The listing builds one solid part. Answer for the finished solid, in the listing's coordinates (mm). A direction names the side the tool comes from. Give positions to 0.01 mm unless a question says otherwise; leave off trailing zeros. Order: outer loops, then holes, each group sorted by start corner. A loop starts at its lowest first (then second) coordinate and runs counter-clockwise, first axis right, second up. Notation, with made-up numbers: (-32, -37.75) - (5, -37.75) arc R23 cw to (5, -18.75) - close; hole circle Ø11 at (45.25, -35.5). An arc over 180 degrees is marked (long way). Answer as a JSON object with one key per item and string values. Group by question number.
Q1. The mould has two halves that part along X. Classify faces 5 (the face through (-10.084, 0.105, 17.68)), 6 (the face through (0.094, -0.424, 11.241)), 7 (the face through (0.588, 9.755, 18.163)): released by +X, released by -X, zero draft, split by the parting line, or undercut.
Q2. A cutting plane is placed at D-D, the plane x = 3.5. Give the vertices of the cut face in (y, z), and give its area (3 significant figures).
Q3. For faces 1 (the face through (12.34, 0.1, 48.11)), 2 (the face through (-8.5, 0, 5)), 3 (the face through (-0.531, 17.36, 20.162)), 4 (the face through (8.5, 0, 5)), determine the directions among +Z, -Z, +X, -X, +Y, -Y from which every point of the face is accessible in a straight line to the end or side of a thin tool.
Q4. A cutting plane is placed at C-C, the plane z = 22.5. Give the vertices of the cut face in (x, y).
Q5. A cutting plane is placed at A-A, the plane z = 33. Give the vertices of the cut face in (x, y).
Q6. Given pin 1 (7 mm diameter, centred on y = 2.5, z = 7, fed in from -X); pin 2 (8.5 mm diameter, centred on x = -4.5, z = 33.5, fed in from +Y); pin 3 (1 mm diameter, centred on x = -6.5, y = 17, fed in from -Z); pin 4 (10 mm diameter, centred on y = -3, z = 4, fed in from +X), each flat-ended and moving along its own axis, determine where each tip first touches the part or whether it passes through.
Q7. Consider line 1 (Y direction, x = 0, z = 3); line 2 (X direction, y = -4, z = 39); line 3 (X direction, y = 25, z = 38). Determine where each line is inside the solid, lowest interval first.
from build123d import *

# Parameters (mm, degrees)
ESQUISSE1_W                    = 17
ESQUISSE1_H                    = 15
BOSS_EXTRU_1_DEPTH             = 20
TROUS_DE_CENTRAGE_5_0MM1_D     = 5
TROUS_DE_CENTRAGE_5_0MM1_DEPTH = 10
TROUS_DE_CENTRAGE_5_0MM1_TIP   = 1.5021515475689007
BOSS_EXTRU_2_DEPTH             = 20
BOSS_EXTRU_3_START             = 15
BOSS_EXTRU_3_DEPTH             = 15
CONG_1_R                       = 19.999999999999996
CONG_2_R                       = 1


with BuildPart() as part:
    # Esquisse1 → Boss.-Extru.1 (new body)
    with BuildSketch(Plane.XY):
        Rectangle(ESQUISSE1_W, ESQUISSE1_H)
    extrude(amount=BOSS_EXTRU_1_DEPTH)

    # Trous de centrage Ø5.0mm1
    with Locations(Plane(origin=(0, 0, 0), x_dir=(-1, 0, 0), z_dir=(0, 0, -1))):
        with Locations((0, 0)):
            Hole(TROUS_DE_CENTRAGE_5_0MM1_D / 2, depth=TROUS_DE_CENTRAGE_5_0MM1_DEPTH)
            with Locations((0, 0, -(TROUS_DE_CENTRAGE_5_0MM1_DEPTH + TROUS_DE_CENTRAGE_5_0MM1_TIP / 2))):  # 118° drill point
                Cone(0, TROUS_DE_CENTRAGE_5_0MM1_D / 2, TROUS_DE_CENTRAGE_5_0MM1_TIP, mode=Mode.SUBTRACT)

    # Esquisse4 → Boss.-Extru.2 (add)
    with BuildSketch(Plane(origin=(0, 7.499999999999998, 0), x_dir=(1, 0, 0), z_dir=(0, 1, 0))):
        with BuildLine():
            Line((-17.89553016817328, -48.65475810617763), (-15.56438241627338, -48.65475810617763))
            ThreePointArc((-15.56438241627338, -48.65475810617763), (-6e-16, -20.15475810617762), (15.564382416273377, -48.65475810617763))
            Line((15.564382416273377, -48.65475810617763), (17.895530168173273, -48.65475810617763))
            ThreePointArc((17.895530168173273, -48.65475810617763), (-4.8e-16, -18.154758106177628), (-17.89553016817328, -48.65475810617763))
        make_face()
    extrude(amount=BOSS_EXTRU_2_DEPTH)

    # Esquisse5 → Boss.-Extru.3 (add)
    with BuildSketch(Plane.XZ.offset(-7.499999999999998).offset(BOSS_EXTRU_3_START)):
        with BuildLine():
            Line((-15.564382416273382, 48.65475810617763), (-11.180339887498954, 48.654758106177624))
            ThreePointArc((-11.180339887498954, 48.654758106177624), (-4.49e-15, 23.65475810617762), (11.180339887498954, 48.654758106177624))
            Line((11.180339887498954, 48.654758106177624), (15.564382416273377, 48.65475810617763))
            Line((15.564382416273377, 48.65475810617763), (17.895530168173273, 48.65475810617763))
            ThreePointArc((17.895530168173273, 48.65475810617763), (19.479599424670532, 32.26764559312642), (8.499999999999998, 20))
            Line((8.499999999999998, 20), (-8.49999999999999, 20))
            ThreePointArc((-8.49999999999999, 20), (-19.47959942467054, 32.26764559312641), (-17.89553016817328, 48.65475810617763))
            Line((-17.89553016817328, 48.65475810617763), (-15.564382416273382, 48.65475810617763))
        make_face()
    extrude(amount=-BOSS_EXTRU_3_DEPTH)

    # Congé1
    cong_1_edges = [part.edges().sort_by_distance(p)[0] for p in [
        (-8.500000000000002, -1.78e-15, 20),
        (8.499999999999998, -1.78e-15, 20),
    ]]
    fillet(cong_1_edges, radius=CONG_1_R)

    # Congé2
    cong_2_edges = [part.edges().sort_by_distance(p)[0] for p in [
        (-17.89553016817328, 9.999999999999998, 48.654758106177624),
        (17.895530168173273, 10, 48.65475810617764),
        (15.564382416273379, 17.5, 48.65475810617763),
        (-15.564382416273382, 17.5, 48.65475810617763),
        (11.180339887498956, -1.78e-15, 48.654758106177624),
        (-11.180339887498954, -1.78e-15, 48.654758106177624),
        (-8.500000000000002, -1.78e-15, 0),
        (8.499999999999998, -1.78e-15, 0),
    ]]
    fillet(cong_2_edges, radius=CONG_2_R - 0.0001)  # a hair under: the kernel refuses the full size


solid = part.part
Reply:
{
 "1": {"face 5": "released by -X", "face 6": "undercut", "face 7": "split by the parting line"},
 "2": {"outline": "(-7.5, 0) - (7.5, 0) - (7.5, 18.46) - (27.5, 18.46) - (27.5, 20.49) - (7.5, 20.49) - (7.5, 24.07) - (-7.5, 24.07) - close", "area": "402 mm^2"},
 "3": {"face 1": "+Y, -Y", "face 2": "-Z, -X, +Y, -Y", "face 3": "+Y", "face 4": "-Z, +X, +Y, -Y"},
 "4": {"outline": "(-12.98, -7.5) - (12.98, -7.5) - (12.98, 7.5) - (12.62, 7.5) - (12.62, 27.5) - (9.02, 27.5) - (9.02, 7.5) - (-9.02, 7.5) - (-9.02, 27.5) - (-12.62, 27.5) - (-12.62, 7.5) - (-12.98, 7.5) - close"},
 "5": {"outline": "(-19.7, -7.5) - (-13.89, -7.5) - (-13.89, 7.5) - (-17.61, 7.5) - (-17.61, 27.5) - (-19.7, 27.5) - close; (13.89, -7.5) - (19.7, -7.5) - (19.7, 27.5) - (17.61, 27.5) - (17.61, 7.5) - (13.89, 7.5) - close"},
 "6": {"pin 1": "stops at x = -8.51", "pin 2": "passes through", "pin 3": "stops at z = 19.05", "pin 4": "stops at x = 8.5"},
 "7": {"line 1": "y = -7.5 to -2.5, 2.5 to 7.5", "line 2": "x = -20.5 to -15, 15 to 20.5", "line 3": "x = -20.49 to -18.49, 18.49 to 20.49"}
}
